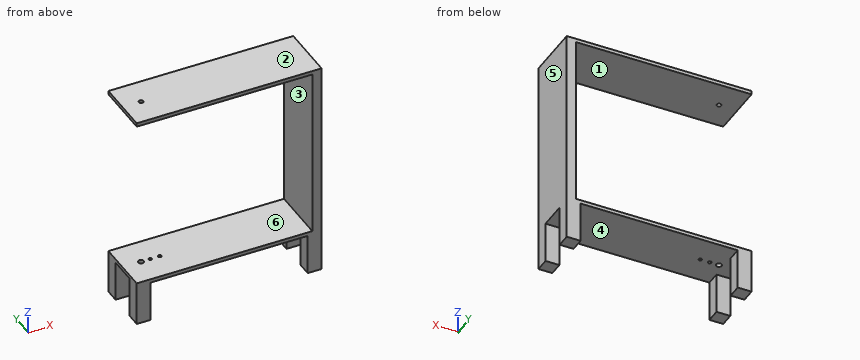
from build123d import *

# Parameters (mm, degrees)
F1_DEPTH = 38.1
F2_R     = 3.048
F3_DEPTH = 246.2286
F4_W     = 19.05
F4_H     = 19.05
F5_DEPTH = 56.134
F6_R     = 2.286
F6_R_2   = 3.81
F6_R_3   = 3.048
F7_DEPTH = 25.4


with BuildPart() as f1:
    # F0 (on Front) → F1 (new body, symmetric)
    with BuildSketch(Plane.XZ):
        Polygon((127, 123.1138), (-127, 123.1138), (-127, 118.0338), (-114.3, 118.0338), (114.3, 118.0338), (114.3, -118.0338), (-114.3, -118.0338), (-127, -118.0338), (-127, -123.1138), (127, -123.1138), align=None)
    extrude(amount=F1_DEPTH, both=True)

    # F2 (on face) → F3 (cut, through all)
    with BuildSketch(Plane.XY.offset(123.1138)):
        with Locations((-101.6, 0)):
            Circle(F2_R)
    extrude(amount=-F3_DEPTH, mode=Mode.SUBTRACT)

    # F4 (on face) → F5 (join)
    with BuildSketch(Plane(origin=(0, 0, -123.1138), x_dir=(1, 0, 0), z_dir=(0, 0, -1))):
        with Locations((-117.475, 28.575)):
            Rectangle(F4_W, F4_H)
        with Locations((-117.475, -28.575)):
            Rectangle(F4_W, F4_H)
        with Locations((117.475, 28.575)):
            Rectangle(F4_W, F4_H)
        with Locations((117.475, -28.575)):
            Rectangle(F4_W, F4_H)
    extrude(amount=F5_DEPTH)

    # F6 (on face) → F7 (cut)
    with BuildSketch(Plane(origin=(0, 0, -123.1138), x_dir=(1, 0, 0), z_dir=(0, 0, -1))):
        with Locations((-88.9, 0)):
            Circle(F6_R)
        with Locations((-75.946, 0)):
            Circle(F6_R)
        with Locations((-101.6, 0)):
            Circle(F6_R_2)
        with Locations((-101.6, 0)):
            Circle(F6_R_3, mode=Mode.SUBTRACT)
    extrude(amount=-F7_DEPTH, mode=Mode.SUBTRACT)


solid = f1.part
Build history of the part. All positions in model axes, mm. Face numbers are marked on the shaded views. A direction names the side the tool comes from. Coordinates: 2 decimals unless noted, no trailing zeros. Write each loop counter-clockwise with the first axis right and the second up, starting at its lowest first coordinate (ties: lowest second). Pieces come first, ordered by that corner, then holes. Notation, with made-up numbers: (7.25, -30.75) -> (47.25, -30.75) arc R7 ccw to (47.25, -23.75) -> close; hole circle Ø8 at (-38, 63). An arc over 180 degrees is marked (long way). Use CSV: the item, a comma, the result in double quotes. Start each with the question number.
Q1. Pull direction X, two halves, no side cores. Call the marked faces 3, 4, 5 and 6: released by +X, released by -X, zero draft, split by the parting line, or undercut.
Q2. Cut at D-D, the plane z = -63.5. List the corners of the cut face in (x, y), then the cut area to 3 significant figures.
Q3. Cut at A-A, the plane x = -44. List the corners of the cut face in (y, z).
Q4. Flat gauge pins, fed straight in: pin 1 Ø10 at (x, y) = (71.5, -30) entering from -Z; pin 2 Ø8 at (y, z) = (-5, -116) entering from -X; pin 3 Ø3 at (y, z) = (-13.5, 75.5) entering from -X. Where does each tip first touch, or does it go through?
Q5. Cut at B-B, the plane z = -155.5. List the corners of the cut face in (x, y), then the cut area to 3 significant figures.
Q6. 3-axis set-ups, long thin cutter, end or side, ignore diameter. For the marked faces 1 and 2: which of +Z, -Z, +X, -X, +Y, -Y reach the whole face in a straight line?
Q7. Drill centre lines: probe 1 along X at (y, z) = (0, -119.2); probe 2 along Z at (x, y) = (-36, 30); probe 3 along Y at (x, z) = (-101, 120). Where is each one in solid material? Low to high.
Q8. Cut at C-C, the plane y = -14.5. List the corners of the cut face in (x, z).
Checked values:
1,face 3,"released by -X"
1,face 4,"undercut"
1,face 5,"released by +X"
1,face 6,"zero draft"
2,outline,"(114.3, -38.1) -> (127, -38.1) -> (127, 38.1) -> (114.3, 38.1) -> close"
2,area,"968 mm²"
3,outline,"(-38.1, -123.11) -> (38.1, -123.11) -> (38.1, -118.03) -> (-38.1, -118.03) -> close; (-38.1, 118.03) -> (38.1, 118.03) -> (38.1, 123.11) -> (-38.1, 123.11) -> close"
4,pin 1,"stops at z = -123.11"
4,pin 2,"stops at x = -127"
4,pin 3,"stops at x = 114.3"
5,outline,"(-127, -38.1) -> (-107.95, -38.1) -> (-107.95, -19.05) -> (-127, -19.05) -> close; (-127, 19.05) -> (-107.95, 19.05) -> (-107.95, 38.1) -> (-127, 38.1) -> close; (107.95, -38.1) -> (127, -38.1) -> (127, -19.05) -> (107.95, -19.05) -> close; (107.95, 19.05) -> (127, 19.05) -> (127, 38.1) -> (107.95, 38.1) -> close"
5,area,"1,450 mm²"
6,face 1,"-X, +Y, -Y"
6,face 2,"+Z, +X, -X, +Y, -Y"
7,probe 1,"x = -127 to -105.41, -97.79 to -91.19, -86.61 to -78.23, -73.66 to 127"
7,probe 2,"z = -123.11 to -118.03, 118.03 to 123.11"
7,probe 3,"y = -38.1 to -2.99, 2.99 to 38.1"
8,outline,"(-127, -123.11) -> (127, -123.11) -> (127, 123.11) -> (-127, 123.11) -> (-127, 118.03) -> (114.3, 118.03) -> (114.3, -118.03) -> (-127, -118.03) -> close"
